Autodesk Inventor part; units mm, degrees
ref_plane "YZ Plane" through (0, 0, 0) normal (1, 0, 0) x (0, 1, 0)
ref_plane "XZ Plane" through (0, 0, 0) normal (0, 1, 0) x (-1, 0, 0)
ref_plane "XY Plane" through (0, 0, 0) normal (0, 0, 1) x (1, 0, 0)
sketch "Esquisse1" plane through (0, 0, 0) normal (0, 0, 1) x (1, 0, 0)
  line L0 (-40, 0) -> (40, 0) construction
  line L1 (-40, -10) -> (40, -10)
  line L2 (40, 10) -> (-40, 10)
  arc A0 (-40, 10) -> (-40, -10) centre (-40, 0) ccw
  arc A1 (40, -10) -> (40, 10) centre (40, 0) ccw
  point P0 (0, 0)
  point P1 (0, 0)
  dimension "d0" = 20
  dimension "d1" = 80
extrude "Extrusion1" add sketch "Esquisse1" along normal blind 6
sketch "Esquisse2" plane through (0, 0, 6) normal (0, 0, 1) x (1, 0, 0)
  line L0 (-37.9704, 0) -> (37.9704, 0) construction
  point P0 (0, 0)
  point P1 (0, 0)
hole "Perçage1" at (-37.9704, 0, 6) at (37.9704, 0, 6) direction (0, 0, -1) diameter 4.2 depth 6 countersink diameter 9 countersink angle 90
sketch "Esquisse3" plane through (0, 0, 0) normal (1, 0, 0) x (0, 1, 0)
  line L0 (10, 6) -> (-10, 6)
  line L1 (10, 6) -> (-18.0536, 33.498)
  line L2 (-10, 0) -> (-10, 6)
  line L3 (-10, 6) -> (-27.8536, 23.5)
  arc A0 (-18.0536, 33.498) -> (-27.8536, 23.5) centre (-22.9536, 28.499) ccw
  circle A1 centre (-22.9536, 28.499) radius 2.6
  point P0 (0, 0)
  dimension "d11" = 14
  dimension "d12" = 5.2
  dimension "d13" = 25
extrude "Extrusion2" add sketch "Esquisse3" along normal mid plane 14
sketch "Esquisse4" plane through (-7, -18.0536, 33.498) normal (0, 0.7, 0.7141) x (1, 0, 0)
  line L0 (11.6, -10) -> (8.4, -10)
  line L1 (8.4, -10) -> (8.4, 10)
  line L2 (8.4, 10) -> (11.6, 10)
  line L3 (11.6, 10) -> (11.6, -10)
  line L4 (0, 0) -> (14, 0)
  line L5 (11.6, -10) -> (8.4, 10) construction
  line L6 (8.4, -10) -> (11.6, 10) construction
  line L7 (7, 0) -> (7, 13.553)
  line L8 (2.4, -10) -> (5.6, -10)
  line L9 (5.6, -10) -> (5.6, 10)
  line L10 (5.6, 10) -> (2.4, 10)
  line L11 (2.4, 10) -> (2.4, -10)
  line L12 (2.4, -10) -> (5.6, 10) construction
  line L13 (5.6, -10) -> (2.4, 10) construction
  point P0 (7, 36.3414)
  point P1 (10, 0)
  point P2 (4, 0)
  dimension "d16" = 3.2
  dimension "d17" = 20
  dimension "d18" = 1.4
extrude "Extrusion3" cut sketch "Esquisse4" along normal through all both and the other way through all
sketch "Esquisse5" plane through (-7, 0, 0) normal (-1, 0, 0) x (0, 0, 1)
  circle A0 centre (28.499, -22.9536) radius 2.6 construction
  circle A1 centre (28.499, -22.9536) radius 7
  line L0 (33.498, -18.0536) -> (6, 10) construction
  line L1 (28.499, -18.3348) -> (32.499, -20.6442)
  line L2 (32.499, -20.6442) -> (32.499, -25.263)
  line L3 (32.499, -25.263) -> (28.499, -27.5724)
  line L4 (28.499, -27.5724) -> (24.499, -25.263)
  line L5 (24.499, -25.263) -> (24.499, -20.6442)
  line L6 (24.499, -20.6442) -> (28.499, -18.3348)
  line L7 (28.499, -22.9536) -> (28.499, -18.3348) construction
  point P0 (0, 0)
  dimension "d21" = 8
extrude "Extrusion4" add sketch "Esquisse5" along normal blind 3
properties part number "support_gopro"
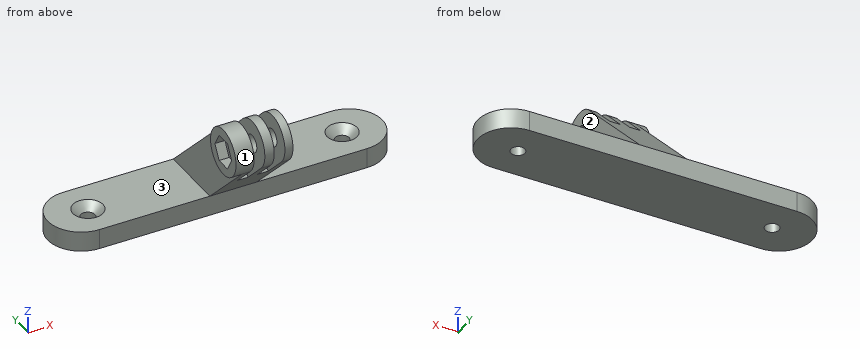
Source: CAD feature listing. Evaluate the final solid. Frame: model axes, mm. Face numbers are marked on the shaded views. A direction names the side the tool comes from. Round coordinates to 2 decimals unless told otherwise and drop trailing zeros. Loops run counter-clockwise (first coordinate to the right, second up) from the corner with the lowest first, then second, coordinate; pieces in that order, holes last. Notation, with made-up numbers: M 29,-37.75 L 78,-37.75 A3 cw 78,-33.75 Z; hole C 46,85.25 d11. An arc over 180 degrees is marked long. Return JSON: item names as keys, results as strings. Group by question number.
1. Section query C-C on x = -2.5. Output: boundary loops of the cut face in (y, z), and give its area (3 significant figures).
2. Section query B-B on y = 0. Output: boundary loops of the cut face in (x, z).
3. Reachability of the marked faces 1, 2 and 3 from +Z, -Z, +X, -X, +Y, -Y: full face, straight path, thin tool, end or side. Return the list, or none.
4. Pin query (flat end, axial travel): pin 1 (5.5 mm diameter, centred on y = -17.5, z = 25.5, fed in from +X); pin 2 (1.5 mm diameter, centred on x = -9, y = -22, fed in from +Z); pin 3 (10 mm diameter, centred on x = 34, y = -1, fed in from +Z). Return the tip coordinate at first contact, or that it passes through.
5. Section query D-D on y = -14. Output: boundary loops of the cut face in (x, z).
6. Material intervals for line 1 along X through (y, z) = (0, 2); line 2 along X through (y, z) = (-23, 22.5); line 3 along X through (y, z) = (-2.5, 10), sorted ascending. Write a range as from..to.
7. Section query A-A on z = 30. State how many separate pieces and enclosed holes the cut face has, and give its area (3 significant figures).
Checks:
{
 "1": {"outline": "M -20.71,16.5 L -10,6 L -10,0 L 10,0 L 10,6 L -10.91,26.5 Z", "area": "430 mm²"},
 "2": {"outline": "M -50,0 L -40.07,0 L -40.07,3.6 L -42.47,6 L -50,6 Z; M -35.87,0 L 35.87,0 L 35.87,3.6 L 33.47,6 L 7,6 L 7,15.8 L -7,15.8 L -7,6 L -33.47,6 L -35.87,3.6 Z; M 40.07,0 L 50,0 L 50,6 L 42.47,6 L 40.07,3.6 Z"},
 "3": {"face 1": "-X", "face 2": "+Z, +X, +Y, -Y", "face 3": "+Z, -X, +Y, -Y"},
 "4": {"pin 1": "stops at x = 7", "pin 2": "stops at z = 35.5", "pin 3": "stops at z = 6"},
 "5": {"outline": "M -7,9.92 L 7,9.92 L 7,29.52 L 4.6,29.52 L 4.6,23.35 L 1.4,23.35 L 1.4,29.52 L -1.4,29.52 L -1.4,23.35 L -4.6,23.35 L -4.6,29.52 L -7,29.52 Z"},
 "6": {"line 1": "x = -50..-40.07, -35.87..35.87, 40.07..50", "line 2": "x = -10..-4.6, -1.4..1.4, 4.6..7", "line 3": "x = -7..7"},
 "7": {"separate pieces": "6", "enclosed holes": "0", "area": "103 mm²"}
}
